from build123d import *

# Parameters (mm, degrees)
SKETCH_1_R      = 4
SKETCH_1_R_2    = 21
EXTRUDE_1_DEPTH = 15


with BuildPart() as part:
    # 草图1 → 凸台-拉伸1 (new body)
    with BuildSketch(Plane.XY):
        Polygon((11, 37.5), (-19, 37.5), (-19, 26.25), (-19, 0), (-19, -37.5), (19, -37.5), (68.446354823, -37.5), (69, 37.5), (19, 37.5), align=None)
        with Locations((-4, -26.25)):
            Circle(SKETCH_1_R, mode=Mode.SUBTRACT)
        with Locations((-4, 26.25)):
            Circle(SKETCH_1_R, mode=Mode.SUBTRACT)
        with Locations((36.5, 0)):
            Circle(SKETCH_1_R_2, mode=Mode.SUBTRACT)
    extrude(amount=EXTRUDE_1_DEPTH)


solid = part.part
Source: CAD feature listing. Evaluate the final solid. Frame: model axes, mm. Round coordinates to 2 decimals unless told otherwise and drop trailing zeros. Write each loop counter-clockwise with the first axis right and the second up, starting at its lowest first coordinate (ties: lowest second). Pieces come first, ordered by that corner, then holes. Notation, with made-up numbers: (-32.75, 79) - (-13.75, 79) arc R35 cw to (-13.75, 117) - close; hole circle Ø2 at (78, 43). An arc over 180 degrees is marked (long way). Use CSV: the item, a comma, the result in double quotes. Start each with the question number.
(1) Cut plane C-C, the plane z = 10. Return loops of the section in (x, y).
(2) Mould query, pull axis Y, two halves, no side actions, for faces 1 (the face through (56.53, 6.31, 7.4)), 2 (the face through (26, 37.5, 7)), 3 (the face through (24, -37.5, 7)), 4 (the face through (15, 1, 15)). Classes: pulls with the +Y half, pulls with the -Y half, needs draft (parallel to the pull), parting line crosses it, or undercut.
(3) Cut plane D-D, the plane y = 26.25. Return loops of the section in (x, z).
(4) First-contact query: pin 1 Ø3 at (x, y) = (-10, 1) entering from -Z; pin 2 Ø12 at (x, y) = (40.5, 10.5) entering from -Z; pin 3 Ø3 at (y, z) = (-6.5, 4) entering from +X. Flat tips, straight axial feed; report the tip coordinate or a pass-through.
(5) Material intervals for probe 1 along Y at (x, z) = (-4, 5.25); probe 2 along Y at (x, z) = (-5, 6); probe 3 along X at (y, z) = (17.5, 10), sorted ascending. Write a range as [from, to].
(6) Cut plane A-A, the plane x = 36.5. Return loops of the section in (y, z).
(7) Cut plane B-B, the plane x = -4. Return loops of the section in (y, z).
Geometry says:
1,outline,"(-19, -37.5) - (68.45, -37.5) - (69, 37.5) - (-19, 37.5) - close; hole circle Ø8 at (-4, -26.25); hole circle Ø8 at (-4, 26.25); hole circle Ø42 at (36.5, 0)"
2,face 1,"undercut"
2,face 2,"pulls with the +Y half"
2,face 3,"pulls with the -Y half"
2,face 4,"needs draft"
3,outline,"(-19, 0) - (-8, 0) - (-8, 15) - (-19, 15) - close; (0, 0) - (68.92, 0) - (68.92, 15) - (0, 15) - close"
4,pin 1,"z = 0"
4,pin 2,"through"
4,pin 3,"x = 68.69"
5,probe 1,"[-37.5, -30.25], [-22.25, 22.25], [30.25, 37.5]"
5,probe 2,"[-37.5, -30.12], [-22.38, 22.38], [30.12, 37.5]"
5,probe 3,"[-19, 24.89], [48.11, 68.85]"
6,outline,"(-37.5, 0) - (-21, 0) - (-21, 15) - (-37.5, 15) - close; (21, 0) - (37.5, 0) - (37.5, 15) - (21, 15) - close"
7,outline,"(-37.5, 0) - (-30.25, 0) - (-30.25, 15) - (-37.5, 15) - close; (-22.25, 0) - (22.25, 0) - (22.25, 15) - (-22.25, 15) - close; (30.25, 0) - (37.5, 0) - (37.5, 15) - (30.25, 15) - close"
